from build123d import *

# Parameters (mm, degrees)
F2_SIZE = 4.99999


# Not quite as in the source:
# - a fillet or chamfer is up to 0.001 mm smaller than in the source, because OpenCascade refuses the exact size
# - a feature names something its author has since deleted; it is built from what else it names


with BuildPart() as f1:
    # F0 (on Top) → F1 (revolve)
    with BuildSketch(Plane.XY):
        Polygon((0, 145), (0, 0), (10, 0), (10, 30), (15, 30), (15, 45), (10, 45), (10, 60), (15, 60), (15, 75), (10, 75), (10, 90), (15, 90), (15, 105), (10, 105), (10, 120), (15, 120), (15, 145), align=None)
    revolve(axis=Axis((0, 72.5, 0), (0, 1, 0)))

    # F2 (size 5 in the source; OpenCascade refuses exactly that, so slightly less here)
    f2_edges = [f1.edges().sort_by_distance(p)[0] for p in [
        (-15, 105, 0),
        (-15, 90, 0),
        (-15, 75, 0),
        (-15, 60, 0),
        (-15, 45, 0),
        (-15, 30, 0),
        (-15, 120, 0),
        (-15, 145, 0),
    ]]
    chamfer(f2_edges, length=F2_SIZE)


solid = f1.part
Can you work these out from the model? Positions are in its coordinate system, mm. A direction names the side the tool comes from. Give positions to 0.01 mm unless a question says otherwise; leave off trailing zeros. Order: outer loops, then holes, each group sorted by start corner. A loop starts at its lowest first (then second) coordinate and runs counter-clockwise, first axis right, second up. Notation, with made-up numbers: (63.25, 69) - (118.25, 69) arc R12 cw to (118.25, 78) - close; hole circle Ø11 at (33, 26.5). An arc over 180 degrees is marked (long way). Write each question's results on one line, items separated by ' | '.
1) On a 3-axis mill with a long thin cutter (end or side, diameter ignored), from which of +Z, -Z, +X, -X, +Y, -Y can I reach the whole of each face in a straight line? I mean faces 1 (the face through (-10.23, 74.76, -0.45)), 2 (the face through (-2.17, 15.21, 9.76)), 3 (the face through (0, 0, 0)). Say none if no direction works.
Final values:
face 1: none | face 2: -Y | face 3: +Z, -Z, +X, -X, -Y
2) I'm going to push flat-ended pins straight in: pin 1 Ø2 at (x, y) = (-1, 44) entering from -Z; pin 2 Ø2 at (x, z) = (11, -8) entering from +Y; pin 3 Ø1.5 at (y, z) = (27.5, 2.5) entering from -X. Where does each tip first touch, or does it pass through?
Final values:
pin 1: stops at z = -11.96 | pin 2: stops at y = 142.4 | pin 3: stops at x = -9.85
3) Suppose I cut it at A-A, the plane z = 12. Give the number of separate pieces and of enclosed holes in the cut face, then the cut area to 3 significant figures.
Final values:
separate pieces: 4 | enclosed holes: 0 | area: 821 mm^2
4) Suppose I cut it at B-B, the plane y = 83.5. Write out the boundary of the cut face in (x, z), then the cut area to 3 significant figures.
Final values:
outline: circle Ø20 at (0, 0) | area: 314 mm^2
5) If we mould it in two halves opening along Y, with no side actions, what happens to faces 4 (the face through (-10.23, 144.76, -0.45)), 5 (the face through (-2.17, 82.6, 9.76)), 6 (the face through (-10.23, 44.76, -0.45)), 7 (the face through (-14.985, 37.535, -0.66))? For each: pulls with the +Y half, pulls with the -Y half, needs draft (parallel to the pull), parting line crosses it, or undercut.
Final values:
face 4: pulls with the +Y half | face 5: undercut | face 6: undercut | face 7: needs draft
6) Please list where these lines run through material, in increasing order: line 1 along Y through (x, z) = (3, -13); line 2 along Y through (x, z) = (0, 13.75); line 3 along Z through (x, y) = (0.25, 133). Write a range as [from, to].
Final values:
line 1: y = [33.34, 41.66], [63.34, 71.66], [93.34, 101.66], [123.34, 141.66] | line 2: y = [33.75, 41.25], [63.75, 71.25], [93.75, 101.25], [123.75, 141.25] | line 3: z = [-15, 15]
